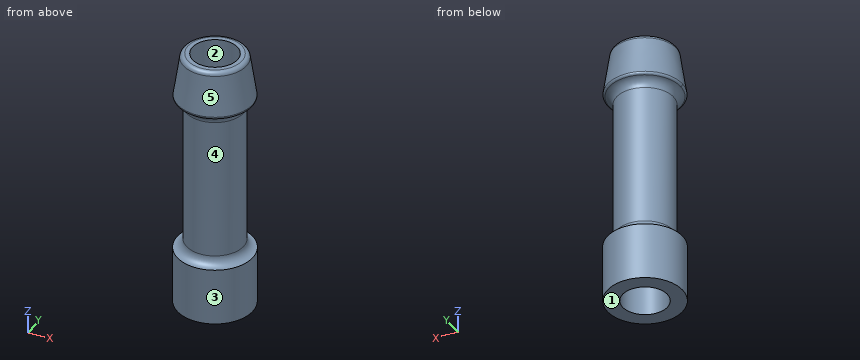
```python
from build123d import *

# Parameters (mm, degrees)
SKETCH1_R           = 4.191
BOSS_EXTRUDE1_DEPTH = 29.21
SKETCH2_R           = 2.5
CUT_EXTRUDE1_START  = -5.08
SKETCH3_R           = 5.08
SKETCH3_R_2         = 3.175
CUT_EXTRUDE1_DEPTH  = 17.78
FILLET1_R           = 1.016
FILLET2_R           = 1.016
CHAMFER1_SIZE       = 5.08
CHAMFER1_SIZE_2     = 0.759211087
FILLET3_R           = 0.254
FILLET4_R           = 0.508


# Some blends are built 0.0001 mm under size
with BuildPart() as part:
    # Sketch1 → Boss-Extrude1 (new body)
    with BuildSketch(Plane.XY):
        with Locations(Location((0, 0, 0), (0, 0, 180))):
            Circle(SKETCH1_R)
    extrude(amount=BOSS_EXTRUDE1_DEPTH)

    # Cut-Sweep1: sweep along a curve in space
    with BuildLine() as cut_sweep1_path:
        Line((0, 0, 29.21), (0, 0, 0))
    # Sketch2 → Cut-Sweep1 (sweep, cut)
    with BuildSketch(Plane.XY.offset(29.21)):
        Circle(SKETCH2_R)
    sweep(path=cut_sweep1_path.line, mode=Mode.SUBTRACT)

    # Sketch3 → Cut-Extrude1 (cut)
    with BuildSketch(Plane.XY.offset(29.21).offset(CUT_EXTRUDE1_START)):
        Circle(SKETCH3_R)
        Circle(SKETCH3_R_2, mode=Mode.SUBTRACT)
    extrude(amount=-CUT_EXTRUDE1_DEPTH, mode=Mode.SUBTRACT)

    # Fillet1
    fillet1_edges = [part.edges().sort_by_distance(p)[0] for p in [
        (-3.175, 0, 6.35),
    ]]
    fillet(fillet1_edges, radius=FILLET1_R - 0.0001)  # a hair under: the kernel refuses the full size

    # Fillet2
    fillet2_edges = [part.edges().sort_by_distance(p)[0] for p in [
        (-3.175, 0, 24.13),
    ]]
    fillet(fillet2_edges, radius=FILLET2_R - 0.0001)  # a hair under: the kernel refuses the full size

    # Chamfer1
    # the kernel refuses this chamfer: 5.08, 0.759211087 mm, written as the material it takes off along each edge
    with BuildSketch(Plane(origin=(0, 0, 29.21), x_dir=(-1, 0, 0), z_dir=(0, 1, 0))) as chamfer1_piece_1:
        Polygon((4.191, -CHAMFER1_SIZE), (4.191 - CHAMFER1_SIZE_2, 0), (4.191, 0), align=None)
    revolve(axis=Axis((0, 0, 29.21), (0, 0, 1)), mode=Mode.SUBTRACT)

    # Fillet3
    fillet3_edges = [part.edges().sort_by_distance(p)[0] for p in [
        (4.191, 0, 24.13),
    ]]
    fillet(fillet3_edges, radius=FILLET3_R)

    # Fillet4
    fillet4_edges = [part.edges().sort_by_distance(p)[0] for p in [
        (3.431788913, 0, 29.21),
    ]]
    fillet(fillet4_edges, radius=FILLET4_R)


solid = part.part
```
For this review, take the finished solid that the model builds, in its own axes (mm). Face numbers are marked on the shaded views. A direction names the side the tool comes from. Coordinates: 2 decimals unless noted, no trailing zeros. Loops run counter-clockwise (first coordinate to the right, second up) from the corner with the lowest first, then second, coordinate; pieces in that order, holes last. Notation, with made-up numbers: (10, 60.5) - (52, 60.5) arc R34 cw to (52, 92.5) - close; hole circle Ø9 at (32, 72.5). An arc over 180 degrees is marked (long way). Use one line per item in the form item = value. Start each with the question number.
1) Take a section at B-B (z = 14.75). State the section outline as (x, y) points (3 decimals), plus the area to 3 significant figures.
2) Draft analysis for pull direction X (two halves, no side actions). For the marked faces 1, 2 and 3, state which applies: released by +X, released by -X, zero draft, split by the parting line, or undercut.
3) For the marked faces 4 and 5, list the 3-axis set-ups (+Z, -Z, +X, -X, +Y, -Y) from which the entire face can be reached by the end or side of a thin tool; tool diameter is ignored.
4) For pin 1 (1.5 mm diameter, centred on x = -3, z = 15, fed in from +Y); pin 2 (3 mm diameter, centred on x = -2, z = 11.5, fed in from -Y); pin 3 (2 mm diameter, centred on x = -2.5, z = 17.5, fed in from +Y), all flat-tipped, find the tip position at first contact; note any pin that passes through.
5) To check wall thickness, follow probe 1 along Y at (x, z) = (0, 9) (3 decimals); probe 2 along Y at (x, z) = (-2, 26.5); probe 3 along X at (y, z) = (1.75, 6.75). State the ranges of each line that lie inside material, in increasing order. Write a range as from..to.
6) Take a section at A-A (z = 25.25). State the section outline as (x, y) points.
From the geometry:
q1.outline = circle Ø6.35 at (0, 0); hole circle Ø5 at (0, 0)
q1.area = 12.0 mm2
q2.face_1 = zero draft
q2.face_2 = undercut
q2.face_3 = split by the parting line
q3.face_4 = none
q3.face_5 = +Z
q4.pin_1 = 2.24
q4.pin_2 = -3.14
q4.pin_3 = 2.8
q5.probe_1 = -3.175..-2.5, 2.5..3.175
q5.probe_2 = -3.27..-1.5, 1.5..3.27
q5.probe_3 = -2.9..-1.79, 1.79..2.9
q6.outline = circle Ø8.05 at (0, 0); hole circle Ø5 at (0, 0)
